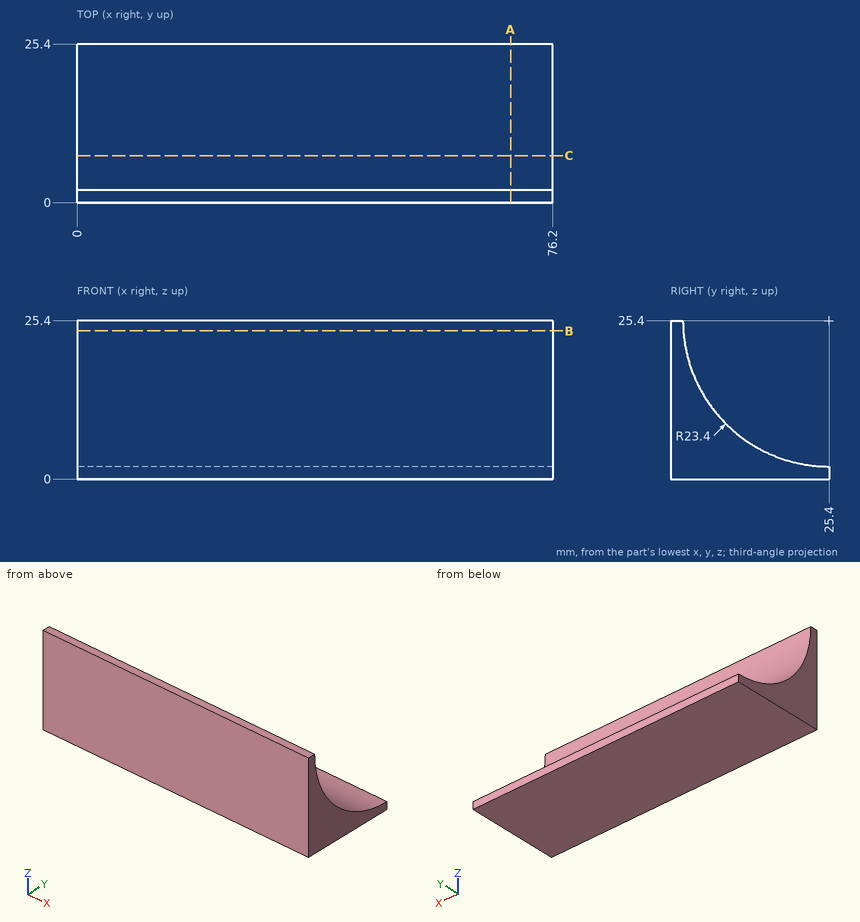
Part print with two shaded views. Sizes in mm from the minimum x, y, z corner. Coordinates: 2 decimals unless noted, no trailing zeros. Write each loop counter-clockwise with the first axis right and the second up, starting at its lowest first coordinate (ties: lowest second). Pieces come first, ordered by that corner, then holes.
1. Drill centre lines: probe 1 along Z at (x, y) = (12, 7.5); probe 2 along Z at (x, y) = (30.5, 13); probe 3 along Y at (x, z) = (43, 14.5). Where is each one in solid material? Low to high.
Answer block:
probe 1: z = 0 to 10.33
probe 2: z = 0 to 5.56
probe 3: y = 0 to 4.69
2. Drop flat-ended pins along their axis: pin 1 (6 mm diameter, centred on x = 37, y = 12, fed in from +Z); pin 2 (1 mm diameter, centred on x = 22.5, y = 9, fed in from +Z); pin 3 (3 mm diameter, centred on x = 57, y = 7, fed in from +Z). Give the stop position or say it passes through.
Answer block:
pin 1: stops at z = 8.71
pin 2: stops at z = 9.22
pin 3: stops at z = 13.09
3. Band-saw the part on B-B, the plane z = 23.75. Give the cut face in (x, y), and give its area (3 significant figures).
Answer block:
outline: (0, 0) - (76.2, 0) - (76.2, 2.06) - (0, 2.06) - close
area: 157 mm2
4. Band-saw the part on A-A, the plane x = 69.5. Give the cut face in (y, z).
Answer block:
outline: (0, 0) - (25.4, 0) - (25.4, 2) arc R23.4 cw to (2, 25.4) - (0, 25.4) - close
5. Band-saw the part on C-C, the plane y = 7.5. Give the cut face in (x, z), and give its area (3 significant figures).
Answer block:
outline: (0, 0) - (76.2, 0) - (76.2, 10.33) - (0, 10.33) - close
area: 787 mm2
